Study the drawing (mm; zero at the part's minimum x, y, z) and answer. Give positions to 0.01 mm unless a question says otherwise; leave off trailing zeros. Order: outer loops, then holes, each group sorted by start corner. A loop starts at its lowest first (then second) coordinate and runs counter-clockwise, first axis right, second up. Notation, with made-up numbers: (6, 76.5) - (56, 76.5) arc R22 cw to (56, 108.5) - close; hole circle Ø2 at (-2.75, -11.75). An arc over 180 degrees is marked (long way). Write each question's results on one line, items separated by ' | '. Start each with the question number.
Q1. Flat-ended cylindrical pins translate along their axes: P1, Ø0.6, axis at x = 25, z = 1, coming from the -Y side; P2, Ø1, axis at y = 18, z = 1.5, coming from the +X side; P3, Ø1, axis at x = 38, z = 1, coming from the +Y side. Find the tip coordinate at first contact, or state that the pin passes through.
Q2. Find section A-A on z = 1.7. Give the vertices of the cut face in (x, y), and give its area (3 significant figures).
Q3. Find section C-C on x = 27.5. Give the vertices of the cut face in (y, z).
Q4. Find the intervals of material crossed by line 1 along X through (y, z) = (2.5, 1.75); line 2 along X through (y, z) = (16, 1); line 3 along Y through (x, z) = (30.5, 0.5), in increasing order. Write a range as from..to.
Q5. Find section B-B on y = 10.75. Give the vertices of the cut face in (x, z), and give its area (3 significant figures).
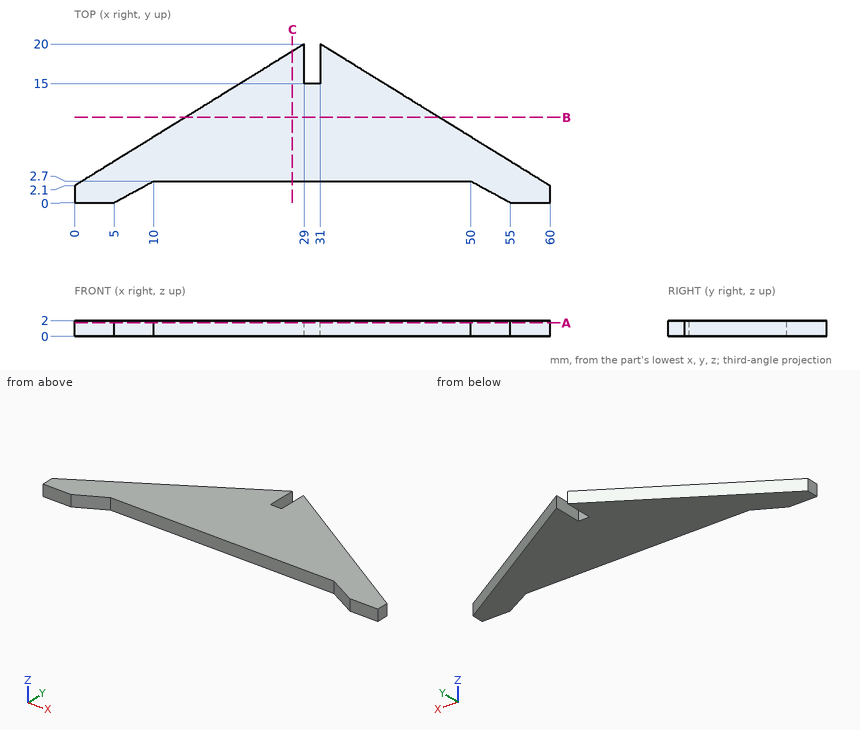
Working result:
1) P1: y = 2.7 | P2: x = 35.05 | P3: y = 15.99
2) outline: (0, 0) - (5, 0) - (10, 2.7) - (50, 2.7) - (55, 0) - (60, 0) - (60, 2.1) - (31, 20) - (31, 15) - (29, 15) - (29, 20) - (0, 2.1) - close | area: 549 mm²
3) outline: (2.7, 0) - (19.07, 0) - (19.07, 2) - (2.7, 2) - close
4) line 1: 0.65..9.63, 50.37..59.35 | line 2: 22.52..29, 31..37.48 | line 3: 2.7..15
5) outline: (14.01, 0) - (45.99, 0) - (45.99, 2) - (14.01, 2) - close | area: 63.9 mm²
